Input: part model. Units: mm. Frame: model coordinates. Face numbers are marked on the shaded views. A direction names the side the tool comes from. Round coordinates to 2 decimals unless told otherwise and drop trailing zeros. Order: outer loops, then holes, each group sorted by start corner. A loop starts at its lowest first (then second) coordinate and runs counter-clockwise, first axis right, second up. Notation, with made-up numbers: (-39.5, -18.5) -> (7.5, -18.5) arc R18 cw to (7.5, 0.5) -> close; hole circle Ø11 at (82.25, 65.5). An arc over 180 degrees is marked (long way). Use a Markdown table: item, result.
from build123d import *

# Parameters (mm, degrees)
SKETCH1_W           = 42
SKETCH1_H           = 42
BOSS_EXTRUDE1_DEPTH = 40
SKETCH2_R           = 11
BOSS_EXTRUDE2_DEPTH = 2
SKETCH3_R           = 2.5
BOSS_EXTRUDE3_DEPTH = 22
SKETCH4_R           = 1.42
CUT_EXTRUDE1_DEPTH  = 5


with BuildPart() as part:
    # Sketch1 → Boss-Extrude1 (new body)
    with BuildSketch(Plane(origin=(0, 0, 0), x_dir=(1, 0, 0), z_dir=(0, 1, 0))):
        Rectangle(SKETCH1_W, SKETCH1_H)
    extrude(amount=BOSS_EXTRUDE1_DEPTH)

    # Sketch2 → Boss-Extrude2 (add)
    with BuildSketch(Plane(origin=(0, 40, 0), x_dir=(1, 0, 0), z_dir=(0, 1, 0))):
        with Locations(Location((0, 0, 0), (0, 0, 90))):
            Circle(SKETCH2_R)
    extrude(amount=BOSS_EXTRUDE2_DEPTH)

    # Sketch3 → Boss-Extrude3 (add)
    with BuildSketch(Plane(origin=(0, 42, 0), x_dir=(1, 0, 0), z_dir=(0, 1, 0))):
        with Locations(Location((0, 0, 0), (0, 0, 270))):
            Circle(SKETCH3_R)
    extrude(amount=BOSS_EXTRUDE3_DEPTH)

    # Sketch4 → Cut-Extrude1 (cut)
    with BuildSketch(Plane(origin=(0, 40, 0), x_dir=(1, 0, 0), z_dir=(0, 1, 0))):
        with Locations(Location((-15.5, 15.5, 0), (0, 0, 270))):
            Circle(SKETCH4_R)
        with Locations(Location((15.5, 15.5, 0), (0, 0, 270))):
            Circle(SKETCH4_R)
        with Locations(Location((15.5, -15.5, 0), (0, 0, 270))):
            Circle(SKETCH4_R)
        with Locations(Location((-15.5, -15.5, 0), (0, 0, 270))):
            Circle(SKETCH4_R)
    extrude(amount=-CUT_EXTRUDE1_DEPTH, mode=Mode.SUBTRACT)


solid = part.part
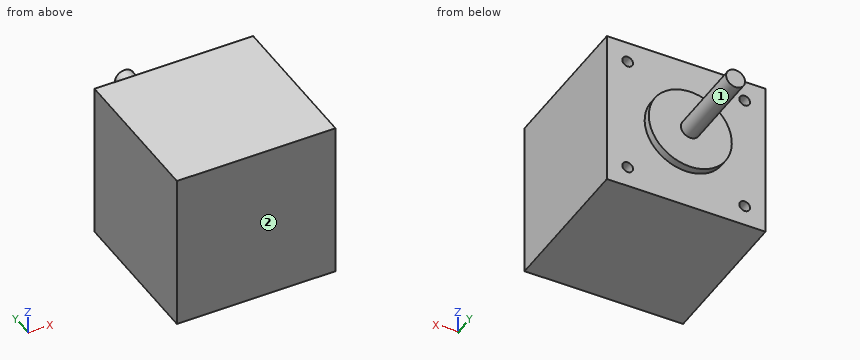
1) Cut plane A-A on x = -15.5. Return loops of the section in (y, z).
Results found:
| item | result |
|---|---|
| outline | (0, -21) -> (40, -21) -> (40, -16.92) -> (35, -16.92) -> (35, -14.08) -> (40, -14.08) -> (40, 14.08) -> (35, 14.08) -> (35, 16.92) -> (40, 16.92) -> (40, 21) -> (0, 21) -> close |
2) Line query: L1, parallel to X at y = 36.7, z = 15.5; L2, parallel to X at y = 37, z = -15; L3, parallel to Y at x = 19.5, z = 13. Output: solid intervals per line, ascending. Write a range as [from, to].
Results found:
| item | result |
|---|---|
| L1 | x = [-21, -16.92], [-14.08, 14.08], [16.92, 21] |
| L2 | x = [-21, -16.83], [-14.17, 14.17], [16.83, 21] |
| L3 | y = [0, 40] |
3) Pin query (flat end, axial travel): pin 1 Ø2.5 at (x, z) = (15.5, 15.5) entering from +Y; pin 2 Ø5 at (y, z) = (53.5, 4.5) entering from -X. Return the tip coordinate at first contact, or that it passes through.
Results found:
| item | result |
|---|---|
| pin 1 | stops at y = 35 |
| pin 2 | stops at x = -1.5 |
4) Set-up query: the marked faces 1 and 2. Return all of +Z, -Z, +X, -X, +Y, -Y with unobstructed straight access to the full face (end or side cutting, diameter ignored); none if empty.
Results found:
| item | result |
|---|---|
| face 1 | +Y |
| face 2 | +Z, -Z, +X, -X, -Y |
5) Cut plane B-B on z = -15.5. Return loops of the section in (x, y).
Results found:
| item | result |
|---|---|
| outline | (-21, 0) -> (21, 0) -> (21, 40) -> (16.92, 40) -> (16.92, 35) -> (14.08, 35) -> (14.08, 40) -> (-14.08, 40) -> (-14.08, 35) -> (-16.92, 35) -> (-16.92, 40) -> (-21, 40) -> close |
6) Cut plane C-C on y = 43. Return loops of the section in (x, z).
Results found:
| item | result |
|---|---|
| outline | circle Ø5 at (0, 0) |
7) Cut plane D-D on x = -7.5. Return loops of the section in (y, z).
Results found:
| item | result |
|---|---|
| outline | (0, -21) -> (40, -21) -> (40, -8.05) -> (42, -8.05) -> (42, 8.05) -> (40, 8.05) -> (40, 21) -> (0, 21) -> close |
